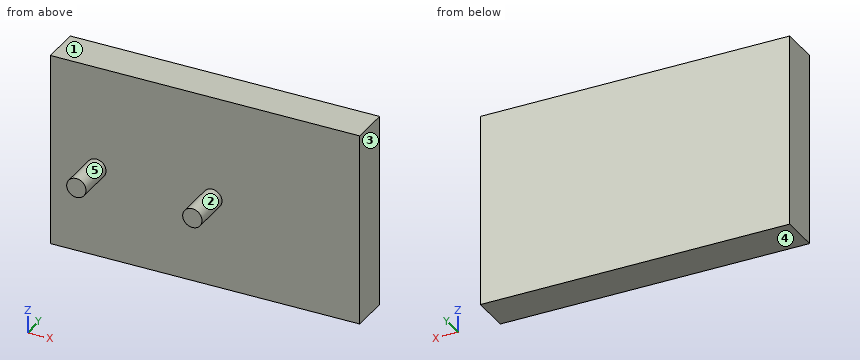
from build123d import *

# Parameters (mm, degrees)
F0_W     = 80
F0_H     = 50
F1_DEPTH = 10
F2_R     = 2.5
F3_DEPTH = 10
F5_DEPTH = 10


with BuildPart() as f1:
    # F0 (on Front) → F1 (new body)
    with BuildSketch(Plane.XZ):
        with Locations((18.104014, 1.864604)):
            Rectangle(F0_W, F0_H)
    extrude(amount=F1_DEPTH)

    # F2 (on face) → F3 (join)
    with BuildSketch(Plane.XZ.offset(10)):
        with Locations((-10, 0)):
            Circle(F2_R)
    extrude(amount=F3_DEPTH)

    # F4 (on face) → F5 (join)
    with BuildSketch(Plane.XZ.offset(10)):
        with BuildLine():
            ThreePointArc((17.5, 0), (20, -2.5), (22.5, 0))
            ThreePointArc((22.5, 0), (20, 2.5), (17.5, 0))
        make_face()
    extrude(amount=F5_DEPTH)


solid = f1.part
Can you work these out from the model? Positions are in its coordinate system, mm. Face numbers are marked on the shaded views. A direction names the side the tool comes from. Give positions to 0.01 mm unless a question says otherwise; leave off trailing zeros. Loops run counter-clockwise (first coordinate to the right, second up) from the corner with the lowest first, then second, coordinate; pieces in that order, holes last. Notation, with made-up numbers: (-2.5, -35) - (20.5, -35) arc R33 cw to (20.5, 2) - close; hole circle Ø1 at (-37, 6). An arc over 180 degrees is marked (long way). Return JSON: item names as keys, results as strings.
1. I want a section at B-B on x = 20. Please give me the cut outline in (y, z).
Output values:
{"outline": "(-20, -2.5) - (-10, -2.5) - (-10, -23.14) - (0, -23.14) - (0, 26.86) - (-10, 26.86) - (-10, 2.5) - (-20, 2.5) - close"}
2. If I drill on line 1 (Y direction, x = 30, z = 14); line 2 (X direction, y = -10.5, z = 1); line 3 (Z direction, x = -10, y = -13.5), over which ranges is the centre line in solid material (lowest first)?
Output values:
{"line 1": "y = -10 to 0", "line 2": "x = -12.29 to -7.71, 17.71 to 22.29", "line 3": "z = -2.5 to 2.5"}
3. We'd pull the mould along X, two halves only. Please class the marked faces 3, 4 and 5: +X half, -X half, draft (parallel to the pull), parting line (faces both ways), or undercut.
Output values:
{"face 3": "+X half", "face 4": "draft", "face 5": "undercut"}
4. I'm going to push a flat-ended pin straight in: pin 1 Ø5 at (x, z) = (40.5, -15.5) entering from -Y. Where does the tip first touch, or does it pass through?
Output values:
{"pin 1": "stops at y = -10"}
5. For the marked faces 1 and 2, which set-ups out of +Z, -Z, +X, -X, +Y, -Y let a thin tool reach every point of the face, with its end or its side?
Output values:
{"face 1": "+Z, +X, -X, +Y, -Y", "face 2": "-Y"}
6. I want a section at D-D on z = 21. Please give me the cut outline in (x, y), and give its area (3 significant figures).
Output values:
{"outline": "(-21.9, -10) - (58.1, -10) - (58.1, 0) - (-21.9, 0) - close", "area": "800 mm²"}
7. I want a section at A-A on z = 1.5. Please give me the cut outline in (x, y).
Output values:
{"outline": "(-21.9, -10) - (-12, -10) - (-12, -20) - (-8, -20) - (-8, -10) - (18, -10) - (18, -20) - (22, -20) - (22, -10) - (58.1, -10) - (58.1, 0) - (-21.9, 0) - close"}
8. I want a section at C-C on y = -15.5. Please give me the cut outline in (x, z), and give its area (3 significant figures).
Output values:
{"outline": "circle Ø5 at (-10, 0); circle Ø5 at (20, 0)", "area": "39.3 mm²"}
